Build history of the part. All positions in model axes, mm. A direction names the side the tool comes from. Round coordinates to 2 decimals unless told otherwise and drop trailing zeros. Loops run counter-clockwise (first coordinate to the right, second up) from the corner with the lowest first, then second, coordinate; pieces in that order, holes last. Notation, with made-up numbers: (-33.75, 49) - (-29.75, 49) arc R8 cw to (-29.75, 60) - close; hole circle Ø1 at (-39, 60). An arc over 180 degrees is marked (long way). Use a Markdown table: item, result.
from build123d import *

# Parameters (mm, degrees)
SKETCH1_W           = 15.9
SKETCH1_H           = 7.95
BOSS_EXTRUDE1_DEPTH = 3.1
SKETCH2_R           = 2.475
BOSS_EXTRUDE2_DEPTH = 1.9
SKETCH3_W           = 12.9
SKETCH3_H           = 4.95
CUT_EXTRUDE1_DEPTH  = 2


with BuildPart() as part:
    # Sketch1 → Boss-Extrude1 (new body)
    with BuildSketch(Plane(origin=(0, 0, 0), x_dir=(1, 0, 0), z_dir=(0, 1, 0))):
        with Locations((-41.303484122, -10.097424035)):
            Rectangle(SKETCH1_W, SKETCH1_H)
    extrude(amount=BOSS_EXTRUDE1_DEPTH)

    # Sketch2 → Boss-Extrude2 (add)
    with BuildSketch(Plane(origin=(0, 3.1, 0), x_dir=(1, 0, 0), z_dir=(0, 1, 0))):
        with Locations(Location((-45.278484122, -10.097424035, 0), (0, 0, 90))):
            Circle(SKETCH2_R)
        with Locations(Location((-37.328484122, -10.097424035, 0), (0, 0, 90))):
            Circle(SKETCH2_R)
    extrude(amount=BOSS_EXTRUDE2_DEPTH)

    # Sketch3 → Cut-Extrude1 (cut)
    with BuildSketch(Plane.XZ):
        with Locations((-41.303484122, 10.097424035)):
            Rectangle(SKETCH3_W, SKETCH3_H)
    extrude(amount=-CUT_EXTRUDE1_DEPTH, mode=Mode.SUBTRACT)


solid = part.part
Q1. Cut at C-C, the plane z = 8.5. List the corners of the cut face in (x, y), plus the area to 3 significant figures.
Results found:
| item | result |
|---|---|
| outline | (-49.25, 0) - (-47.75, 0) - (-47.75, 2) - (-34.85, 2) - (-34.85, 0) - (-33.35, 0) - (-33.35, 3.1) - (-35.44, 3.1) - (-35.44, 5) - (-39.22, 5) - (-39.22, 3.1) - (-43.39, 3.1) - (-43.39, 5) - (-47.17, 5) - (-47.17, 3.1) - (-49.25, 3.1) - close |
| area | 37.9 mm2 |
Q2. Cut at A-A, the plane y = 1.2. List the corners of the cut face in (x, z).
Results found:
| item | result |
|---|---|
| outline | (-49.25, 6.12) - (-33.35, 6.12) - (-33.35, 14.07) - (-49.25, 14.07) - close; hole (-47.75, 7.62) - (-34.85, 7.62) - (-34.85, 12.57) - (-47.75, 12.57) - close |
Q3. Pull direction X, two halves, no side cores. Call faces 1 (the face through (-39.782, 4.037, 10.42)), 2 (the face through (-45, 5, 10)), 3 (the face through (-33.353, 2, 10)), 4 (the face through (-49.253, 2, 10)): pulls with the +X half, pulls with the -X half, needs draft (parallel to the pull), parting line crosses it, or undercut.
Results found:
| item | result |
|---|---|
| face 1 | undercut |
| face 2 | needs draft |
| face 3 | pulls with the +X half |
| face 4 | pulls with the -X half |
Q4. Which spindle directions (+Z, -Z, +X, -X, +Y, -Y) get a long thin tool onto all of the face, cutting with end or side? Do faces 5 (the face through (-34.853, 1, 10)), 6 (the face through (-41, 2, 6.122)), 7 (the face through (-41, 3.1, 10)). Say none if no direction does.
Results found:
| item | result |
|---|---|
| face 5 | -Y |
| face 6 | -Z, +X, -X, +Y, -Y |
| face 7 | +Y |
Q5. Cut at D-D, the plane x = -47.5. List the corners of the cut face in (y, z).
Results found:
| item | result |
|---|---|
| outline | (0, 6.12) - (3.1, 6.12) - (3.1, 9.01) - (5, 9.01) - (5, 11.19) - (3.1, 11.19) - (3.1, 14.07) - (0, 14.07) - (0, 12.57) - (2, 12.57) - (2, 7.62) - (0, 7.62) - close |
Q6. Probe line 1 (Z direction, x = -46, y = 1.4); line 2 (X direction, y = 3.55, z = 10); line 3 (Y direction, x = -36.5, z = 12.5). List the from-to ranges inside material, lowest first.
Results found:
| item | result |
|---|---|
| line 1 | z = 6.12 to 7.62, 12.57 to 14.07 |
| line 2 | x = -47.75 to -42.81, -39.8 to -34.86 |
| line 3 | y = 2 to 3.1 |
Q7. Drop a flat-ended pin along its axis: pin 1 (1.5 mm diameter, centred on x = -44.5, y = 4, fed in from +Z). Give the stop position or say it passes through.
Results found:
| item | result |
|---|---|
| pin 1 | stops at z = 12.57 |
Q8. Cut at B-B, the plane x = -41. List the corners of the cut face in (y, z), plus the area to 3 significant figures.
Results found:
| item | result |
|---|---|
| outline | (0, 6.12) - (3.1, 6.12) - (3.1, 14.07) - (0, 14.07) - (0, 12.57) - (2, 12.57) - (2, 7.62) - (0, 7.62) - close |
| area | 14.7 mm2 |
